Can you work these out from the model? Positions are in its coordinate system, mm. A direction names the side the tool comes from. Give positions to 0.01 mm unless a question says otherwise; leave off trailing zeros. Order: outer loops, then holes, each group sorted by start corner. A loop starts at its lowest first (then second) coordinate and runs counter-clockwise, first axis right, second up. Notation, with made-up numbers: (70.25, 7.25) -> (104.25, 7.25) arc R27 ccw to (104.25, 42.25) -> close; hole circle Ø8 at (75.5, 57). An arc over 180 degrees is marked (long way). Answer as CSV lines item,"result".
```python
from build123d import *

# Parameters (mm, degrees)
SKETCH1_R           = 1.9
BOSS_EXTRUDE1_DEPTH = 1
SKETCH2_R           = 2.940420278
BOSS_EXTRUDE2_DEPTH = 2
CHAMFER1_SIZE       = 0.5
SKETCH3_R           = 1
CUT_EXTRUDE1_DEPTH  = 4
CHAMFER2_SIZE       = 0.1


with BuildPart() as part:
    # Sketch1 → Boss-Extrude1 (new body)
    with BuildSketch(Plane(origin=(0, 0, 0), x_dir=(1, 0, 0), z_dir=(0, 1, 0))):
        with Locations(Location((0, 0, 0), (0, 0, 270))):
            Circle(SKETCH1_R)
    extrude(amount=BOSS_EXTRUDE1_DEPTH)

    # Sketch2 → Boss-Extrude2 (add)
    with BuildSketch(Plane(origin=(0, 1, 0), x_dir=(1, 0, 0), z_dir=(0, 1, 0))):
        with Locations(Location((0, 0, 0), (0, 0, 270))):
            Circle(SKETCH2_R)
    extrude(amount=BOSS_EXTRUDE2_DEPTH)

    # Chamfer1
    chamfer1_edges = [part.edges().sort_by_distance(p)[0] for p in [
        (0, 3, -2.940420278),
    ]]
    chamfer(chamfer1_edges, length=CHAMFER1_SIZE)

    # Sketch3 → Cut-Extrude1 (cut)
    with BuildSketch(Plane(origin=(0, 3, 0), x_dir=(1, 0, 0), z_dir=(0, 1, 0))):
        with Locations(Location((0, 0, 0), (0, 0, 270))):
            Circle(SKETCH3_R)
    extrude(amount=-CUT_EXTRUDE1_DEPTH, mode=Mode.SUBTRACT)

    # Chamfer2
    chamfer2_edges = [part.edges().sort_by_distance(p)[0] for p in [
        (0, 3, -1),
    ]]
    chamfer(chamfer2_edges, length=CHAMFER2_SIZE)


solid = part.part
```
Item 1: Imagine slicing it at C-C, the plane y = 1.7. Please give me the cut outline in (x, z).
Numbers:
outline,"circle Ø5.88 at (0, 0); hole circle Ø2 at (0, 0)"
Item 2: For pin 1 (1.6 mm diameter, centred on x = 0, z = 0, fed in from -Y), with a flat end and sliding along its axis, tell me the tip position at first contact or that it passes through.
Numbers:
pin 1,"passes through"
Item 3: For faces 1 (the cylindrical face through (-0.728, 0.493, 1.755)), 2 (the flat face through (-1, 3, 1)), which set-ups out of +Z, -Z, +X, -X, +Y, -Y let a thin tool reach every point of the face, with its end or its side?
Numbers:
face 1,"-Y"
face 2,"+Z, -Z, +X, -X, +Y"
Item 4: We'd pull the mould along Z, two halves only. Please class faces 3 (the cylindrical face through (-1, 1, 0)), 4 (the cylindrical face through (-1.789, 1.74, -2.333)), 5 (the flat face through (-1, 0, 1)): released by +Z, released by -Z, zero draft, split by the parting line, or undercut.
Numbers:
face 3,"undercut"
face 4,"split by the parting line"
face 5,"zero draft"
Item 5: Imagine slicing it at B-B, the plane z = 0. Please give me the cut outline in (x, y), then the cut area to 3 significant figures.
Numbers:
outline,"(-2.94, 1) -> (-1.9, 1) -> (-1.9, 0) -> (-1, 0) -> (-1, 2.9) -> (-1.1, 3) -> (-2.44, 3) -> (-2.94, 2.5) -> close; (1, 0) -> (1.9, 0) -> (1.9, 1) -> (2.94, 1) -> (2.94, 2.5) -> (2.44, 3) -> (1.1, 3) -> (1, 2.9) -> close"
area,"9.30 mm²"
Item 6: Please list where these lines run through material, in increasing order: line 1 along X through (y, z) = (1.45, 0); line 2 along X through (y, z) = (0.95, 0).
Numbers:
line 1,"x = -2.94 to -1, 1 to 2.94"
line 2,"x = -1.9 to -1, 1 to 1.9"
Item 7: Imagine slicing it at A-A, the plane x = 0. Please give me the cut outline in (y, z).
Numbers:
outline,"(0, -1.9) -> (1, -1.9) -> (1, -2.94) -> (2.5, -2.94) -> (3, -2.44) -> (3, -1.1) -> (2.9, -1) -> (0, -1) -> close; (0, 1) -> (2.9, 1) -> (3, 1.1) -> (3, 2.44) -> (2.5, 2.94) -> (1, 2.94) -> (1, 1.9) -> (0, 1.9) -> close"
